Design review of the part built by this model. Coordinates are the model's own, in mm. Face numbers are marked on the shaded views. Round coordinates to 2 decimals unless told otherwise and drop trailing zeros. Loops run counter-clockwise (first coordinate to the right, second up) from the corner with the lowest first, then second, coordinate; pieces in that order, holes last. Notation, with made-up numbers: M 76.25,37.5 L 102.25,37.5 A13 cw 102.25,51.5 Z; hole C 72,-7 d4. An arc over 180 degrees is marked long. Answer as CSV lines item,"result". Start each with the question number.
from build123d import *

# Parameters (mm, degrees)
F3_R     = 8.89
F4_DEPTH = 25.4
F5_R     = 1.778


with BuildPart() as f2:
    # F0 (on Front) → F2 (revolve)
    with BuildSketch(Plane.XZ):
        with BuildLine():
            Line((-3.81, 0), (0, 0))
            Line((0, 0), (3.81, 0))
            Line((3.81, 0), (3.81, 20.86))
            ThreePointArc((3.81, 20.86), (0, 17.05), (-3.81, 20.86))
            Line((-3.81, 20.86), (-3.81, 0))
        make_face()
        Polygon((-4.81, 0), (-3.81, 0), (-3.81, 20.86), (-3.81, 22.86), (-4.81, 22.86), align=None)
        Polygon((3.81, 20.86), (3.81, 0), (4.81, 0), (4.81, 22.86), (3.81, 22.86), align=None)
    revolve(axis=Axis((-0.3435998224, 0, 0), (1, 0, 0)))

    # F3 (on face) → F4 (cut)
    with BuildSketch(Plane(origin=(-4.81, 0, 0), x_dir=(0, -1, 0), z_dir=(-1, 0, 0))):
        Circle(F3_R)
    extrude(amount=-F4_DEPTH, mode=Mode.SUBTRACT)

    # F5
    f5_edges = [f2.edges().sort_by_distance(p)[0] for p in [
        (4.81, 8.89, 0),
        (-4.81, 8.89, 0),
    ]]
    fillet(f5_edges, radius=F5_R)


solid = f2.part
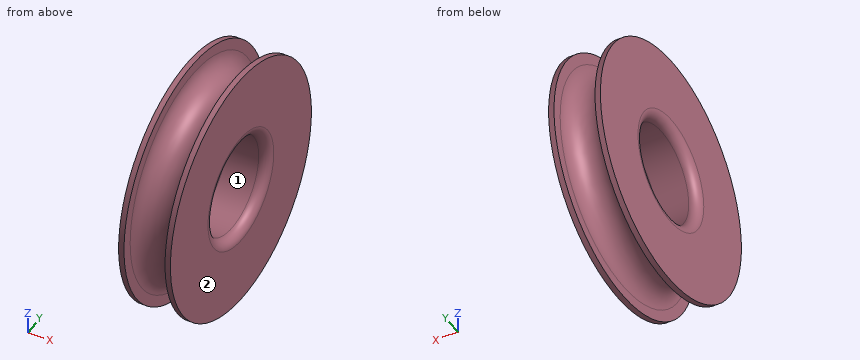
Item 1: Insertion check: pin 1 Ø2 at (x, z) = (2, 5.5) entering from +Y; pin 2 Ø5 at (x, y) = (-1, -6) entering from +Z; pin 3 Ø1 at (x, y) = (-3, 1) entering from -Z; pin 4 Ø23 at (y, z) = (2, -7) entering from +X. Each pin has a flat end and moves straight along its axis. Give the tip position at first contact, or say it passes through.
Item 2: The part is to be moulded in two halves that separate along Y. For the marked faces 1 and 2, say which applies: +Y half, -Y half, draft (parallel to the pull), parting line (faces both ways), or undercut.
Item 3: To check wall thickness, follow line 1 (Y direction, x = -1.5, z = -1.5); line 2 (X direction, y = 0.5, z = 20); line 3 (Z direction, x = -1, y = 0). State the ranges of each line that lie inside material, in increasing order.
Item 4: Consider section A-A, the plane z = 0. Write out the cut boundary in (x, y), then the cut area to 3 significant figures.
Item 5: Consider section C-C, the plane x = 1.75. Write out the cut boundary in (y, z), then the cut area to 3 significant figures.
Found:
1,pin 1,"stops at y = 17.71"
1,pin 2,"stops at z = 18.45"
1,pin 3,"stops at z = -19.33"
1,pin 4,"stops at x = 4.81"
2,face 1,"undercut"
2,face 2,"draft"
3,line 1,"y = -17.29 to -8.76, 8.76 to 17.29"
3,line 2,"x = -4.81 to -3.71, 3.71 to 4.81"
3,line 3,"z = -17.18 to -8.89, 8.89 to 17.18"
4,outline,"M -4.81,-22.86 L -3.81,-22.86 L -3.81,-20.86 A3.81 cw 3.81,-20.86 L 3.81,-22.86 L 4.81,-22.86 L 4.81,-10.67 A1.78 ccw 3.03,-8.89 L -3.03,-8.89 A1.78 ccw -4.81,-10.67 Z; M -4.81,10.67 A1.78 ccw -3.03,8.89 L 3.03,8.89 A1.78 ccw 4.81,10.67 L 4.81,22.86 L 3.81,22.86 L 3.81,20.86 A3.81 cw -3.81,20.86 L -3.81,22.86 L -4.81,22.86 Z"
4,area,"190 mm^2"
5,outline,"C 0,0 d34.95; hole C 0,0 d17.78"
5,area,"711 mm^2"
